Work out the finished part from the listing and answer in its coordinate system (mm). Face numbers are marked on the shaded views. Round coordinates to 2 decimals unless told otherwise and drop trailing zeros. Write each loop counter-clockwise with the first axis right and the second up, starting at its lowest first coordinate (ties: lowest second). Pieces come first, ordered by that corner, then holes. Notation, with made-up numbers: M -15.5,-39.5 L 2.5,-39.5 A17 ccw 2.5,-6.5 Z; hole C 86.25,31.25 d2. An arc over 180 degrees is marked long. One line per item, written item: value. Start each with the question number.
Q1. Given pin 1 Ø10 at (x, z) = (-6, 0.5) entering from +Y; pin 2 Ø4 at (x, y) = (-8.5, 12) entering from -Z; pin 3 Ø6 at (y, z) = (6, -6) entering from +X, each flat-ended and moving along its own axis, determine where each tip first touches the part or whether it passes through.
Q2. Find section A-A (x = 0). Write down the section's boundary in (y, z), and give its area (3 significant figures).
Q3. Find section B-B (y = 9). Write down the section's boundary in (x, z) (1 decimal), and give its area (3 significant figures).
Q4. Consider probe 1 along Z at (x, y) = (0, 0.95); probe 2 along X at (y, z) = (13.2, 0). Determine where each line is inside the solid, lowest interval first.
Q5. The mould has two halves that part along X. Classify the marked faces 1 and 2: released by +X, released by -X, zero draft, split by the parting line, or undercut.
Q6. Find section C-C (y = 3.75). Write down the section's boundary in (x, z).
Autodesk Inventor part; units mm, degrees
ref_plane "Work Plane1" through (0, 11.9, 0) normal (0, 1, 0) x (1, 0, 0)
ref_plane "YZ Plane" through (0, 0, 0) normal (1, 0, 0) x (0, 1, 0)
ref_plane "XZ Plane" through (0, 0, 0) normal (0, 1, 0) x (-1, 0, 0)
sketch "Sketch1" plane through (0, 0, 0) normal (0, 1, 0) x (-1, 0, 0)
  circle A0 centre (0, 0) radius 6.8
  circle A1 centre (0, 0) radius 7.8
  dimension "d0" = 13.6
  dimension "d1" = 15.6
extrude "Extrusion1" add sketch "Sketch1" along normal blind 1.9
sketch "Sketch2" plane through (0, 1.9, 0) normal (0, 1, 0) x (1, 0, 0)
  circle A0 centre (0, 0) radius 7.8
  dimension "d20" = 15.6
ref_plane "Work Plane1" through (0, 11.9, 0) normal (0, 1, 0) x (1, 0, 0)
sketch "Sketch3" plane through (0, 11.9, 0) normal (0, 1, 0) x (1, 0, 0)
  circle A0 centre (0, 0) radius 16
  dimension "d6" = 32
loft "Loft1" add profiles "Sketch3" section 1 edges at (7.8, 1.9, 0)
sketch "Sketch4" plane through (0, 1.9, 0) normal (0, -1, 0) x (1, 0, 0)
  circle A0 centre (0, 0) radius 5.75
  dimension "d12" = 11.5
sketch "Sketch5" plane through (0, 11.9, 0) normal (0, 1, 0) x (1, 0, 0)
  circle A0 centre (0, 0) radius 14.5
  dimension "d13" = 29
loft "Loft2" cut profiles "Sketch4", "Sketch5"
sketch "Sketch6" plane through (0, 11.9, 0) normal (0, 1, 0) x (1, 0, 0)
  circle A0 centre (0, 0) radius 14.5
  circle A1 centre (0, 0) radius 16
  dimension "d21" = 32
  dimension "d22" = 29
extrude "Extrusion2" add sketch "Sketch6" along normal blind 2
properties part number "Widefield_LightShield_Cone"
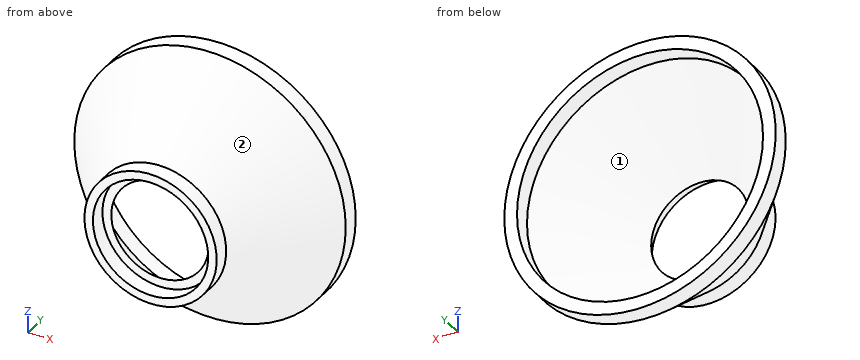
The answers:
1. pin 1: y = 7.92
1. pin 2: z = -14.62
1. pin 3: x = 12.53
2. outline: M 0,-7.8 L 1.9,-7.8 L 11.9,-16 L 13.9,-16 L 13.9,-14.5 L 11.9,-14.5 L 1.9,-5.75 L 1.9,-6.8 L 0,-6.8 Z; M 0,6.8 L 1.9,6.8 L 1.9,5.75 L 11.9,14.5 L 13.9,14.5 L 13.9,16 L 11.9,16 L 1.9,7.8 L 0,7.8 Z
2. area: 45.3 mm2
3. outline: C 0,0 d27.2; hole C 0,0 d23.9
3. area: 133 mm2
4. probe 1: -7.8 to -6.8, 6.8 to 7.8
4. probe 2: -16 to -14.5, 14.5 to 16
5. face 1: undercut
5. face 2: split by the parting line
6. outline: C 0,0 d18.63; hole C 0,0 d14.74
